Autodesk Inventor part; units mm, degrees
ref_plane "Work Plane1" through (-30.1251, 9, -4) normal (1, 0, 0) x (0, 0, -1)
ref_plane "Work Plane2" through (-23.3752, 9, -4) normal (1, 0, 0) x (0, 0, -1)
ref_plane "YZ Plane" through (0, 0, 0) normal (1, 0, 0) x (0, 1, 0)
sketch "Sketch1" plane through (0, 0, 0) normal (0, 1, 0) x (-1, 0, 0)
  line L0 (0, 0) -> (35.5, 0)
  line L1 (35.5, 0) -> (35.5, -90)
  line L2 (35.5, -90) -> (0, -90)
  line L3 (0, -90) -> (0, 0)
  dimension "d0" = 35.5
  dimension "d1" = 90
extrude "Extrusion1" add sketch "Sketch1" along normal blind 9
sketch "Sketch3" plane through (0, 0, 0) normal (0, -1, 0) x (1, 0, 0)
  circle A0 centre (-10, -25) radius 3.25 construction
  line L0 (0, 0) -> (-35.5, 0)
  line L1 (-35.5, 0) -> (-35.5, -90)
  line L2 (-11.6286, -27.8125) -> (-13.25, -24.9958)
  line L3 (-13.25, -24.9958) -> (-11.6214, -22.1833)
  line L4 (-11.6214, -22.1833) -> (-8.3714, -22.1875)
  line L5 (-8.3714, -22.1875) -> (-6.75, -25.0042)
  line L6 (-6.75, -25.0042) -> (-8.3786, -27.8167)
  line L7 (-8.3786, -27.8167) -> (-11.6286, -27.8125)
  line L8 (0, -90) -> (0, 0)
  dimension "d15" = 6.5
  dimension "d16" = 25
  dimension "d26" = 10
extrude "Extrusion3" cut sketch "Sketch3" against normal blind 5
sketch "Sketch5" plane through (0, 9, 0) normal (0, 1, 0) x (1, 0, 0)
  line L0 (0, 0) -> (0, 90)
  line L1 (-35.5, 0) -> (0, 0)
  circle A0 centre (-10, 25) radius 1.7
  dimension "d36" = 3.4
  dimension "d37" = 25
extrude "Extrusion4" cut sketch "Sketch5" against normal through all
sketch "Sketch6" plane through (0, 9, 0) normal (0, 1, 0) x (1, 0, 0)
  line L0 (-32.5, 4) -> (-27.7502, 4)
  line L1 (-27.7502, 4) -> (-27.7502, 29.4)
  line L2 (-27.7502, 29.4) -> (-32.5, 29.4)
  line L3 (-32.5, 29.4) -> (-32.5, 4)
  line L4 (-35.5, 0) -> (0, 0)
  line L5 (-35.5, 90) -> (-35.5, 0)
  line L6 (-25.7502, 4) -> (-21.0002, 4)
  line L7 (-21.0002, 4) -> (-21.0002, 16.7)
  line L8 (-21.0002, 16.7) -> (-25.7502, 16.7)
  line L9 (-25.7502, 16.7) -> (-25.7502, 4)
  line L10 (0, 0) -> (0, 90) construction
  line L11 (-35.5, 90) -> (0, 90)
  line L12 (0, 0) -> (-20, 0) construction
  line L13 (-20, 0) -> (-20, 90) construction
  line L14 (-20, 90) -> (0, 90) construction
  line L15 (0, 90) -> (0, 0)
  circle A0 centre (-23.3752, 41.7) radius 1.7
  circle A1 centre (-30.125, 41.7) radius 1.7
  circle A2 centre (-30.125, 49.7) radius 1.7
  circle A3 centre (-23.3752, 49.7) radius 1.7
  dimension "d43" = 4.7498
  dimension "d44" = 25.4
  dimension "d45" = 4
  dimension "d46" = 3
  dimension "d47" = 4.75
  dimension "d48" = 2
  dimension "d49" = 20
  dimension "d50" = 3.4
  dimension "d90" = 3.4
  dimension "d91" = 5.375
  dimension "d92" = 3.4
  dimension "d93" = 8
  dimension "d94" = 3.4
  dimension "d99" = 40.3
extrude "Extrusion5" cut sketch "Sketch6" against normal through all contours L3 L2 L1 L0 | L9 L8 L7 L6 | A0 | A1 | A2 | A3
sketch "Sketch7" plane through (0, 0, 0) normal (0, -1, 0) x (1, 0, 0)
  circle A0 centre (-23.3752, -41.7) radius 1.7
  circle A1 centre (-23.3752, -41.7) radius 3.25 construction
  line L0 (-23.3752, -38.45) -> (-20.5606, -40.075)
  line L1 (-20.5606, -40.075) -> (-20.5606, -43.325)
  line L2 (-20.5606, -43.325) -> (-23.3752, -44.95)
  line L3 (-23.3752, -44.95) -> (-26.1898, -43.325)
  line L4 (-26.1898, -43.325) -> (-26.1898, -40.075)
  line L5 (-26.1898, -40.075) -> (-23.3752, -38.45)
  line L6 (0, 0) -> (-35.5, 0)
  circle A2 centre (-30.125, -41.7) radius 3.25 construction
  line L7 (-35.5, 0) -> (-35.5, -90)
  line L8 (-30.1645, -44.9498) -> (-32.9591, -43.2907)
  line L9 (-32.9591, -43.2907) -> (-32.9196, -40.0409)
  line L10 (-32.9196, -40.0409) -> (-30.0855, -38.4502)
  line L11 (-30.0855, -38.4502) -> (-27.2909, -40.1093)
  line L12 (-27.2909, -40.1093) -> (-27.3304, -43.3591)
  line L13 (-27.3304, -43.3591) -> (-30.1645, -44.9498)
  dimension "d88" = 6.5
  dimension "d54" = 6.5
  dimension "d87" = 41.7
  dimension "d89" = 5.375
extrude "Extrusion6" cut sketch "Sketch7" against normal blind 5
sketch "Sketch8" plane through (-35.5, 0, -90) normal (-1, 0, 0) x (0, 0, 1)
  circle A0 centre (79.65, 4.5) radius 1.4605
  line L0 (0, 9) -> (90, 9)
  line L1 (90, 0) -> (90, 9)
  circle A1 centre (66.95, 4.5) radius 1.4605
  dimension "d57" = 2.921
  dimension "d58" = 4.5
  dimension "d59" = 10.35
  dimension "d103" = 2.921
  dimension "d104" = 4.5
  dimension "d105" = 12.7
hole "Hole1" at (-35.5, 4.5, -10.35) at (-35.5, 4.5, -23.05) direction (1, 0, 0) diameter 2.921 depth 21 counterbore diameter 3.4 counterbore depth 1.5
sketch "Sketch9" plane through (-21.0002, 9, -16.7) normal (-1, 0, 0) x (0, 0, 1)
  circle A0 centre (6.35, -4.5) radius 1.4605
  circle A1 centre (6.35, -4.5) radius 2.54
  point P0 (16.7, -9)
  dimension "d67" = 5.08
extrude "Extrusion7" add sketch "Sketch9" along normal blind 0.2032
sketch "Sketch10" plane through (-27.7502, 9, -29.4) normal (-1, 0, 0) x (0, 0, 1)
  circle A0 centre (6.35, -4.5) radius 1.7
  circle A1 centre (6.35, -4.5) radius 2.54
  circle A2 centre (19.05, -4.5) radius 2.54
  circle A3 centre (19.05, -4.5) radius 2.54
  circle A4 centre (19.05, -4.5) radius 1.7
  point P0 (29.4, -9)
  dimension "d70" = 5.08
  dimension "d106" = 3.4
extrude "Extrusion8" add sketch "Sketch10" along normal blind 0.2032
sketch "Sketch11" plane through (-25.7502, 9, -4) normal (1, 0, 0) x (0, 0, -1)
  circle A0 centre (6.35, -4.5) radius 1.7
  circle A1 centre (6.35, -4.5) radius 2.54
  point P0 (-4, -9)
  dimension "d73" = 5.08
extrude "Extrusion9" add sketch "Sketch11" along normal blind 0.2032
sketch "Sketch12" plane through (-32.5, 9, -4) normal (1, 0, 0) x (0, 0, -1)
  circle A0 centre (6.35, -4.5) radius 1.7
  circle A1 centre (6.35, -4.5) radius 2.54
  circle A2 centre (19.05, -4.5) radius 1.4605
  circle A3 centre (19.05, -4.5) radius 2.54
  circle A4 centre (19.05, -4.5) radius 1.7
  point P0 (-4, -9)
  dimension "d76" = 5.08
  dimension "d107" = 5.08
  dimension "d108" = 3.4
extrude "Extrusion10" add sketch "Sketch12" along normal blind 0.2032 contours A1 | A3
sketch "Sketch14" plane through (0, 0, -90) normal (0, 0, -1) x (-1, 0, 0)
  circle A0 centre (18, 4.5) radius 2.25
  line L0 (35.5, 0) -> (0, 0)
  line L1 (0, 0) -> (0, 9)
  dimension "d82" = 4.5
  dimension "d83" = 4.5
  dimension "d84" = 18
extrude "Extrusion11" cut sketch "Sketch14" against normal blind 41
sketch "Sketch15" plane through (0, 9, 0) normal (0, 1, 0) x (1, 0, 0)
  circle A0 centre (-30.125, 49.7) radius 1.7
  circle A1 centre (-30.125, 49.7) radius 3.25 construction
  circle A2 centre (-23.3752, 49.7) radius 1.7
  circle A3 centre (-23.3752, 49.7) radius 3.25 construction
  line L0 (-30.125, 52.95) -> (-27.3104, 51.325)
  line L1 (-27.3104, 51.325) -> (-27.3104, 48.075)
  line L2 (-27.3104, 48.075) -> (-30.125, 46.45)
  line L3 (-30.125, 46.45) -> (-32.9396, 48.075)
  line L4 (-32.9396, 48.075) -> (-32.9396, 51.325)
  line L5 (-32.9396, 51.325) -> (-30.125, 52.95)
  line L6 (-23.3752, 52.95) -> (-20.5606, 51.325)
  line L7 (-20.5606, 51.325) -> (-20.5606, 48.075)
  line L8 (-20.5606, 48.075) -> (-23.3752, 46.45)
  line L9 (-23.3752, 46.45) -> (-26.1898, 48.075)
  line L10 (-26.1898, 48.075) -> (-26.1898, 51.325)
  line L11 (-26.1898, 51.325) -> (-23.3752, 52.95)
  point P0 (0, 0)
  dimension "d95" = 6.5
  dimension "d96" = 6.5
extrude "Extrusion12" cut sketch "Sketch15" against normal blind 5
ref_plane "Work Plane1" through (-30.1251, 9, -4) normal (1, 0, 0) x (0, 0, -1)
ref_plane "Work Plane2" through (-23.3752, 9, -4) normal (1, 0, 0) x (0, 0, -1)
sketch "Sketch18" plane through (0, 0, 0) normal (1, 0, 0) x (0, 0, -1)
  circle A0 centre (4, 4.5) radius 1.45
  line L0 (0, 0) -> (0, 9)
  line L1 (0, 9) -> (90, 9)
  line L2 (90, 0) -> (0, 0)
  circle A1 centre (9, 4.5) radius 1.45
  circle A2 centre (14, 4.5) radius 1.45
  circle A3 centre (19, 4.5) radius 1.45
  circle A4 centre (24, 4.5) radius 1.45
  circle A5 centre (29, 4.5) radius 1.45
  circle A6 centre (34, 4.5) radius 1.45
  circle A7 centre (39, 4.5) radius 1.45
  circle A8 centre (44, 4.5) radius 1.45
  circle A9 centre (49, 4.5) radius 1.45
  dimension "d116" = 2.9
  dimension "d117" = 4
  dimension "d118" = 4.5
  dimension "d119" = 9
  dimension "d122" = 5
extrude "Extrusion13" cut sketch "Sketch18" against normal blind 6
equation "\"d118\" = 0.5 * d119"
properties part number "Front fixed top coupler"
Part model, mm, in its own coordinate system. A direction names the side the tool comes from. Coordinates: 2 decimals unless noted, no trailing zeros. Order: outer loops, then holes, each group sorted by start corner. A loop starts at its lowest first (then second) coordinate and runs counter-clockwise, first axis right, second up. Notation, with made-up numbers: M -24.75,88.5 L -0.75,88.5 A24 ccw -0.75,103.5 Z; hole C -20.5,25 d8. An arc over 180 degrees is marked long. Use a Markdown table: item, result.
(1) Probe L1, parallel to Z at x = -26.95, y = 4.5; L2, parallel to Z at x = -16, y = 4.5; L3, parallel to Y at x = -4.35, z = -19. List the from-to ranges inside material, lowest first.
A:
| item | result |
|---|---|
| L1 | z = -90 to -24.51, -21.59 to -11.81, -8.89 to 0 |
| L2 | z = -49 to -24.51, -21.59 to -11.81, -8.89 to 0 |
| L3 | y = 0 to 3.05, 5.95 to 9 |
(2) Flat gauge pins, fed straight in: pin 1 (5 mm diameter, centred on x = -18, y = 4.5, fed in from +Z); pin 2 (1 mm diameter, centred on y = 3.5, z = -10.5, fed in from -X); pin 3 (2 mm diameter, centred on y = 4.5, z = -10.35, fed in from -X); pin 4 (1.4 mm diameter, centred on y = 4, z = -24, fed in from +X). Where does each tip first touch, or does it go through?
A:
| item | result |
|---|---|
| pin 1 | stops at z = 0 |
| pin 2 | stops at x = -34 |
| pin 3 | stops at x = -14.5 |
| pin 4 | stops at x = -6 |
(3) Tool access for faces 5 (the flat face through (-32.94, 7, -50)), 6 (the flat face through (-26.19, 2, -42)), 7 (the cylindrical face through (-2.958, 3.945, -35.339)): list every direction of +Z, -Z, +X, -X, +Y, -Y with a clear straight run to the whole face (end or side of a thin tool).
A:
| item | result |
|---|---|
| face 5 | +Y |
| face 6 | -Y |
| face 7 | +X |
(4) Pull direction Z, two halves, no side cores. Call faces 1 (the flat face through (-28.698, 6.535, -47.274)), 2 (the cylindrical face through (-21.805, 7.028, -41.049)), 3 (the flat face through (-18, 0, -44)), 4 (the flat face through (-18, 7, -90)): released by +Z, released by -Z, zero draft, split by the parting line, or undercut.
A:
| item | result |
|---|---|
| face 1 | undercut |
| face 2 | undercut |
| face 3 | zero draft |
| face 4 | released by -Z |
(5) Cut at D-D on z = -14.5. Write the cut outline in (x, y), then the cut area to 3 significant figures.
A:
| item | result |
|---|---|
| outline | M -35.5,0 L -32.5,0 L -32.5,9 L -35.5,9 Z; M -27.75,0 L -25.75,0 L -25.75,9 L -27.75,9 Z; M -21,0 L 0,0 L 0,3.14 L -6,3.14 L -6,5.86 L 0,5.86 L 0,9 L -21,9 Z |
| area | 218 mm^2 |
(6) Cut at A-A on x = -3. State how many separate pieces and enclosed holes the cut face has, then the cut area to 3 significant figures.
A:
| item | result |
|---|---|
| separate pieces | 1 |
| enclosed holes | 10 |
| area | 744 mm^2 |
(7) Cut at C-C on x = -18. Write the cut outline in (y, z).
A:
| item | result |
|---|---|
| outline | M 0,-90 L 2.25,-90 L 2.25,-49 L 6.75,-49 L 6.75,-90 L 9,-90 L 9,0 L 0,0 Z; hole C 4.5,-23.05 d2.92; hole C 4.5,-10.35 d2.92 |
(8) Cut at B-B on z = -74.5. Write the cut outline in (x, y), then the cut area to 3 significant figures.
A:
| item | result |
|---|---|
| outline | M -35.5,0 L 0,0 L 0,9 L -35.5,9 Z; hole C -18,4.5 d4.5 |
| area | 304 mm^2 |
